Verification items for this drawing (mm, ordinates from the low corner). A direction names the side the tool comes from. Give positions to 0.01 mm unless a question says otherwise; leave off trailing zeros. Order: outer loops, then holes, each group sorted by start corner. A loop starts at its lowest first (then second) coordinate and runs counter-clockwise, first axis right, second up. Notation, with made-up numbers: M -34,43 L 7,43 A8 cw 7,51 Z; hole C 76,-22 d5. An arc over 180 degrees is marked long. Return JSON: item names as keys, results as strings. Group by question number.
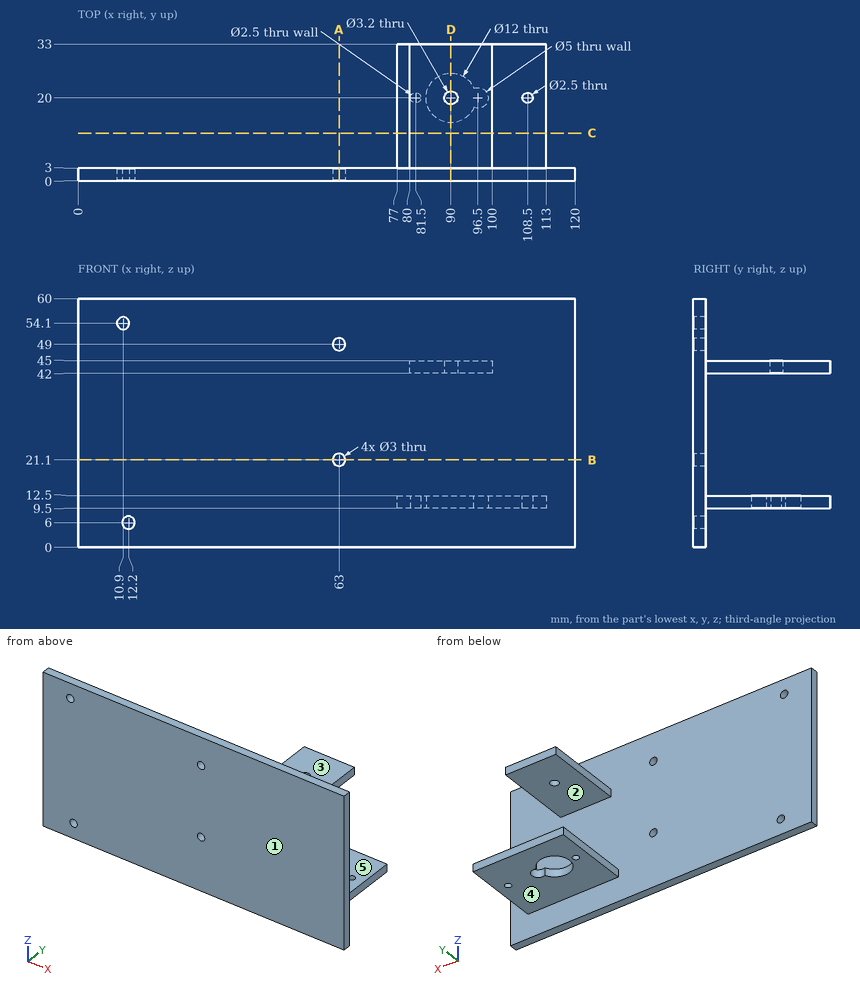
1) Material ranges on line 1 along Z through (x, y) = (63, 1.2); line 2 along X through (y, z) = (0.75, 6); line 3 along X through (y, z) = (20, 43), recorded low to high.
2) Sectioned sample at B-B on z = 21.1. Record the boundary of the cut face in (x, y).
3) Depth check by flat-ended pin: P1, Ø3.5, axis at y = 18.5, z = 43, coming from the -X side; P2, Ø9, axis at x = 103.5, y = 18.5, coming from the -Z side; P3, Ø2.5, axis at x = 10.9, z = 54.1, coming from the -Y side; P4, Ø3, axis at x = 100.5, y = 23.5, coming from the +Z side. Enter the tip coordinate at first touch or a pass-through.
4) Sectioned sample at C-C on y = 11.5. Record the boundary of the cut face in (x, z).
5) Sectioned sample at D-D on x = 90. Record the boundary of the cut face in (y, z).
6) Sectioned sample at A-A on x = 63. Record the boundary of the cut face in (y, z).
7) Tool access check on the marked faces 4 and 5. Record the directions out of +Z, -Z, +X, -X, +Y, -Y that give a thin tool (end or side, any length) a straight path to the whole face; none if there is none.
8) Release check for a two-part mould opening along Z. For the marked faces 1, 2 and 3 record: released by +Z, released by -Z, zero draft, split by the parting line, or undercut.
Reply:
{
 "1": {"line 1": "0 to 19.6, 22.6 to 47.5, 50.5 to 60", "line 2": "0 to 10.7, 13.7 to 120", "line 3": "80 to 88.4, 91.6 to 100"},
 "2": {"outline": "M 0,0 L 61.5,0 L 61.5,3 L 0,3 Z; M 64.5,0 L 120,0 L 120,3 L 64.5,3 Z"},
 "3": {"P1": "x = 80", "P2": "z = 9.5", "P3": "through", "P4": "z = 45"},
 "4": {"outline": "M 77,9.5 L 113,9.5 L 113,12.5 L 77,12.5 Z; M 80,42 L 100,42 L 100,45 L 80,45 Z"},
 "5": {"outline": "M 0,0 L 3,0 L 3,9.5 L 14,9.5 L 14,12.5 L 3,12.5 L 3,42 L 18.4,42 L 18.4,45 L 3,45 L 3,60 L 0,60 Z; M 21.6,42 L 33,42 L 33,45 L 21.6,45 Z; M 26,9.5 L 33,9.5 L 33,12.5 L 26,12.5 Z"},
 "6": {"outline": "M 0,0 L 3,0 L 3,19.6 L 0,19.6 Z; M 0,22.6 L 3,22.6 L 3,47.5 L 0,47.5 Z; M 0,50.5 L 3,50.5 L 3,60 L 0,60 Z"},
 "7": {"face 4": "-Z, +X, -X, +Y", "face 5": "+X, -X, +Y"},
 "8": {"face 1": "zero draft", "face 2": "undercut", "face 3": "released by +Z"}
}
